The model under review builds one solid part; all positions refer to its coordinate system, in mm. Round coordinates to 2 decimals unless told otherwise and drop trailing zeros. Write each loop counter-clockwise with the first axis right and the second up, starting at its lowest first coordinate (ties: lowest second). Pieces come first, ordered by that corner, then holes. Notation, with made-up numbers: (34, 31) -> (58, 31) arc R8 ccw to (58, 41) -> close; hole circle Ø8 at (46.25, 15.5). An arc over 180 degrees is marked (long way). Return JSON: item names as keys, results as strings. Group by question number.
1. For line 1 along X through (y, z) = (11.5, -109), list the stretches that pass through material, from the lowest coordinate up. Write a range as from..to.
2. Take a section at B-B, the plane z = -145. Write out the cut boundary in (x, y).
3. Take a section at A-A, the plane y = -8. Write out the cut boundary in (x, z).
4. Take a section at C-C, the plane x = -6.5. Write out the cut boundary in (y, z).
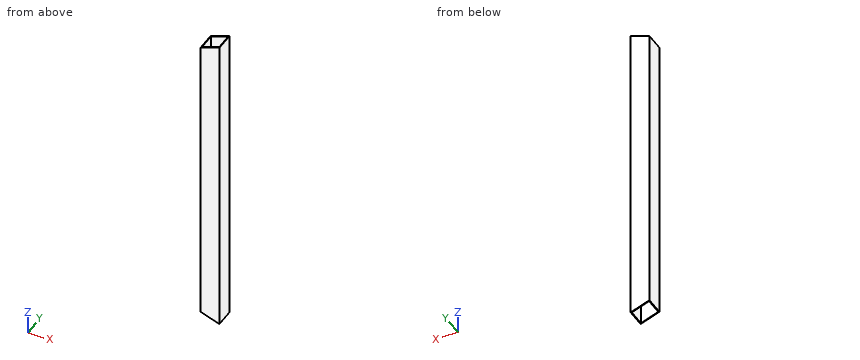
Autodesk Inventor part; units mm, degrees
ref_plane "YZ Plane" through (0, 0, 0) normal (1, 0, 0) x (0, 1, 0)
ref_plane "XZ Plane" through (0, 0, 0) normal (0, 1, 0) x (-1, 0, 0)
ref_plane "XY Plane" through (0, 0, 0) normal (0, 0, 1) x (1, 0, 0)
sketch "Sketch1" plane through (0, 0, 0) normal (0, 0, 1) x (1, 0, 0)
  line L0 (-25.4, 25.4) -> (25.4, 25.4)
  line L1 (25.4, 25.4) -> (25.4, -25.4)
  line L2 (25.4, -25.4) -> (-25.4, -25.4)
  line L3 (-25.4, -25.4) -> (-25.4, 25.4)
  line L4 (23.2918, 23.2918) -> (-23.2918, 23.2918)
  line L5 (-23.2918, 23.2918) -> (-23.2918, -23.2918)
  line L6 (-23.2918, -23.2918) -> (23.2918, -23.2918)
  line L7 (23.2918, -23.2918) -> (23.2918, 23.2918)
  point P0 (0, 0)
  point P1 (0, 25.4)
  point P2 (23.2918, 0)
  dimension "d0" = 50.8
  dimension "d1" = 50.8
  dimension "d2" = 2.1082
extrude "Extrusion1" add sketch "Sketch1" along normal mid plane 838.2
sketch "Sketch2" plane through (-25.4, 25.4, 419.1) normal (0, 1, 0) x (1, 0, 0)
  line L0 (50.8, 0) -> (109.4588, 0) construction
  line L1 (50.0284, 838.2) -> (109.4588, 838.2) construction
  line L2 (50.8, 0) -> (0, 18.4897)
  line L3 (50.8, 0) -> (104.8602, 0) construction
  line L4 (0, 18.4897) -> (0, 0)
  line L5 (0, 0) -> (50.8, 0)
  line L6 (50.0284, 838.2) -> (109.4588, 838.2) construction
  line L7 (0, 838.2) -> (50.0284, 838.2)
  line L8 (0, 838.2) -> (0, 0)
  line L9 (50.0284, 838.2) -> (0, 819.9912)
  line L10 (50.0284, 838.2) -> (103.2675, 838.2) construction
  line L11 (0, 819.9912) -> (0, 838.2)
  point P0 (25.4, 419.1)
  dimension "d7" = 160
  dimension "d11" = 160
extrude "Extrusion2" cut sketch "Sketch2" against normal through all
properties part number "TV mount center"
Output:
{
 "1": {"line 1": "x = -25.4..-23.29, 23.29..25.4"},
 "2": {"outline": "(-25.4, -25.4) -> (25.4, -25.4) -> (25.4, 25.4) -> (-25.4, 25.4) -> close; hole (-23.29, -23.29) -> (23.29, -23.29) -> (23.29, 23.29) -> (-23.29, 23.29) -> close"},
 "3": {"outline": "(-25.4, -400.89) -> (-23.29, -401.66) -> (-23.29, 401.38) -> (-25.4, 400.61) -> close; (23.29, -418.61) -> (24.63, -419.1) -> (25.4, -419.1) -> (25.4, 419.1) -> (23.29, 418.33) -> close"},
 "4": {"outline": "(-25.4, -407.77) -> (-23.29, -407.77) -> (-23.29, 407.49) -> (-25.4, 407.49) -> close; (23.29, -407.77) -> (25.4, -407.77) -> (25.4, 407.49) -> (23.29, 407.49) -> close"}
}
